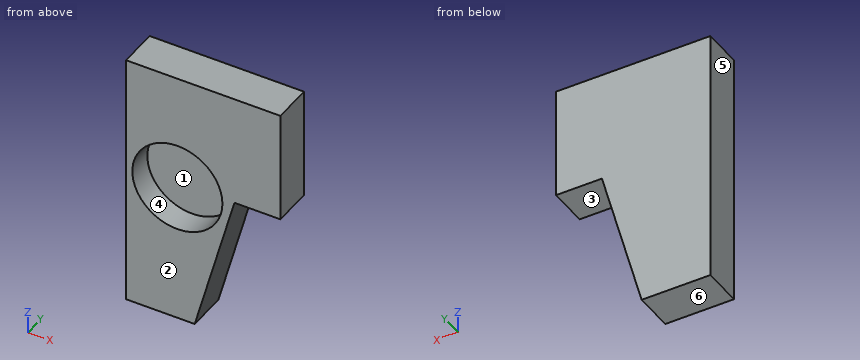
```python
from build123d import *

# Parameters (mm, degrees)
F1_DEPTH = 15.759194
F2_R     = 17.831749
F3_DEPTH = 10


with BuildPart() as f1:
    # F0 (on Front) → F1 (new body)
    with BuildSketch(Plane.XZ):
        Polygon((0, -28.000414), (27.195573, -28.000414), (42.920023, 30.085534), (61.09336, 30.085534), (61.09336, 74.423328), (0, 74.423328), align=None)
    extrude(amount=F1_DEPTH)

    # F2 (on face) → F3 (cut)
    with BuildSketch(Plane.XZ.offset(15.759194)):
        with Locations((20.327643, 27.81529)):
            Circle(F2_R)
    extrude(amount=-F3_DEPTH, mode=Mode.SUBTRACT)


solid = f1.part
```
Design review of the part built by this model. Coordinates are the model's own, in mm. Face numbers are marked on the shaded views. A direction names the side the tool comes from. Coordinates: 2 decimals unless noted, no trailing zeros. Write each loop counter-clockwise with the first axis right and the second up, starting at its lowest first coordinate (ties: lowest second). Pieces come first, ordered by that corner, then holes. Notation, with made-up numbers: M 46.25,25 L 66.25,25 A11 cw 66.25,35 Z; hole C 68.5,9.5 d9. An arc over 180 degrees is marked long. Answer as a JSON object with one key per item and string values.
Item 1: Machinability: for the marked faces 1, 2 and 3, which of the approach directions +Z, -Z, +X, -X, +Y, -Y give a long, thin tool a straight path to every point of the face, cutting with its end or side? Answer none if there is none.
Outcome:
{"face 1": "-Y", "face 2": "+Z, -Z, +X, -X, -Y", "face 3": "-Z, +X, +Y, -Y"}
Item 2: Add section A-A, the plane y = -6.75. Give the boundary of the cut face in (x, z), and give its area (3 significant figures).
Outcome:
{"outline": "M 0,-28 L 27.2,-28 L 42.92,30.09 L 61.09,30.09 L 61.09,74.42 L 0,74.42 Z; hole C 20.33,27.82 d35.66", "area": "3,750 mm²"}
Item 3: Draft analysis for pull direction X (two halves, no side actions). For the marked faces 4, 5 and 6, state which applies: pulls with the +X half, pulls with the -X half, needs draft (parallel to the pull), parting line crosses it, or undercut.
Outcome:
{"face 4": "undercut", "face 5": "pulls with the -X half", "face 6": "needs draft"}
Item 4: Wall thickness on probe 1 along X at (y, z) = (-7.25, 28.5); probe 2 along Z at (x, y) = (13, -7); probe 3 along Z at (x, y) = (12.5, -14.5): over which ranges is each line inside the solid? List them lowest first.
Outcome:
{"probe 1": "0 to 2.51, 38.15 to 42.49", "probe 2": "-28 to 11.56, 44.07 to 74.42", "probe 3": "-28 to 11.79, 43.84 to 74.42"}
Item 5: Add section B-B, the plane y = -2.5. Give the boundary of the cut face in (x, z), and give its area (3 significant figures).
Outcome:
{"outline": "M 0,-28 L 27.2,-28 L 42.92,30.09 L 61.09,30.09 L 61.09,74.42 L 0,74.42 Z", "area": "4,750 mm²"}
Item 6: Add section C-C, the plane x = 9.5. Give the boundary of the cut face in (y, z), and give its area (3 significant figures).
Outcome:
{"outline": "M -15.76,-28 L 0,-28 L 0,74.42 L -15.76,74.42 L -15.76,41.98 L -5.76,41.98 L -5.76,13.65 L -15.76,13.65 Z", "area": "1,330 mm²"}
Item 7: Insertion check: pin 1 Ø18 at (x, z) = (15, 33) entering from -Y. The pin has a flat end and moves straight along its axis. Give the tip position at first contact, or say it passes through.
Outcome:
{"pin 1": "y = -5.76"}
Item 8: Add section D-D, the plane z = 18. Give the boundary of the cut face in (x, y).
Outcome:
{"outline": "M 0,-15.76 L 5.44,-15.76 L 5.44,-5.76 L 35.21,-5.76 L 35.21,-15.76 L 39.65,-15.76 L 39.65,0 L 0,0 Z"}
